from build123d import *

# Parameters (mm, degrees)
F0_W      = 45
F0_H      = 27
F0_R      = 1.5
F0_H_2    = 12
F1_DEPTH  = 8
F2_DEPTH  = 28
F3_R      = 1.5
F4_DEPTH  = 10
F5_DEPTH  = 8
F6_W      = 31
F6_H      = 12
F7_DEPTH  = 20
F8_SIZE2  = 19.5
F8_SIZE   = 20
F9_SIZE2  = 7.5
F9_SIZE   = 20
F11_DEPTH = 19.501
F12_DEPTH = 3
F13_R     = 7.7732339674
F14_DEPTH = 3
F16_DEPTH = 10
F17_DEPTH = 8
F18_R     = 1.5
F19_DEPTH = 16


with BuildPart() as f1:
    # F0 (on Top) → F1 (new body)
    with BuildSketch(Plane.XY):
        Rectangle(F0_W, F0_H)
        with Locations((-10, -10)):
            Circle(F0_R, mode=Mode.SUBTRACT)
        with Locations((10, -10)):
            Circle(F0_R, mode=Mode.SUBTRACT)
        with Locations((-10, 10)):
            Circle(F0_R, mode=Mode.SUBTRACT)
        with Locations((10, 10)):
            Circle(F0_R, mode=Mode.SUBTRACT)
        with Locations((0, 19.5)):
            Rectangle(F0_W, F0_H_2)
        with Locations((-10, 22)):
            Circle(F0_R, mode=Mode.SUBTRACT)
        with Locations((10, 22)):
            Circle(F0_R, mode=Mode.SUBTRACT)
    extrude(amount=F1_DEPTH)

    # F0 (on Top) → F2 (join)
    with BuildSketch(Plane.XY):
        with Locations((0, 19.5)):
            Rectangle(F0_W, F0_H_2)
        with Locations((-10, 22)):
            Circle(F0_R, mode=Mode.SUBTRACT)
        with Locations((10, 22)):
            Circle(F0_R, mode=Mode.SUBTRACT)
    extrude(amount=-F2_DEPTH)

    # F3 (on face) → F4 (cut)
    with BuildSketch(Plane(origin=(0, 0, -28), x_dir=(1, 0, 0), z_dir=(0, 0, -1))):
        Polygon((-7.25, -20.4122867597), (-10, -18.8245735195), (-12.75, -20.4122867597), (-12.75, -23.5877132403), (-12.75, -25.5), (-7.25, -25.5), (-7.25, -23.5877132403), align=None)
        with Locations((-10, -22)):
            Circle(F3_R, mode=Mode.SUBTRACT)
        Polygon((7.25, -23.5877132403), (7.25, -25.5), (12.75, -25.5), (12.75, -23.5877132403), (12.75, -20.4122867597), (10, -18.8245735195), (7.25, -20.4122867597), align=None)
        with Locations((10, -22)):
            Circle(F3_R, mode=Mode.SUBTRACT)
    extrude(amount=-F4_DEPTH, mode=Mode.SUBTRACT)

    # F3 (on face) → F5 (join)
    with BuildSketch(Plane(origin=(0, 0, -28), x_dir=(1, 0, 0), z_dir=(0, 0, -1))):
        Polygon((7.25, -23.5877132403), (7.25, -25.5), (12.75, -25.5), (12.75, -23.5877132403), (12.75, -20.4122867597), (10, -18.8245735195), (7.25, -20.4122867597), align=None)
        with Locations((10, -22)):
            Circle(F3_R, mode=Mode.SUBTRACT)
        Polygon((-7.25, -20.4122867597), (-10, -18.8245735195), (-12.75, -20.4122867597), (-12.75, -23.5877132403), (-12.75, -25.5), (-7.25, -25.5), (-7.25, -23.5877132403), align=None)
        with Locations((-10, -22)):
            Circle(F3_R, mode=Mode.SUBTRACT)
    extrude(amount=-F5_DEPTH)

    # F6 (on face) → F7 (join)
    with BuildSketch(Plane.XY.offset(8)):
        Polygon((-22.5, 25.5), (-22.5, -13.5), (-15.5, -13.5), (-15.5, -6), (-15.5, 6), (-15.5, 25.5), align=None)
        Rectangle(F6_W, F6_H)
        Polygon((15.5, 6), (15.5, -6), (15.5, -13.5), (22.5, -13.5), (22.5, 25.5), (15.5, 25.5), align=None)
    extrude(amount=F7_DEPTH)

    # F8
    f8_edges = [f1.edges().sort_by_distance(p)[0] for p in [
        (-19, 25.5, 28),
        (19, 25.5, 28),
    ]]
    f8_side = f1.faces().sort_by_distance((0, 25.5, -5.719915))[0]
    chamfer(f8_edges, length=F8_SIZE, length2=F8_SIZE2, reference=f8_side)

    # F9
    f9_edges = [f1.edges().sort_by_distance(p)[0] for p in [
        (19, -13.5, 28),
        (-19, -13.5, 28),
    ]]
    f9_side = f1.faces().sort_by_distance((-21.97, -13.5, 14))[0]
    chamfer(f9_edges, length=F9_SIZE, length2=F9_SIZE2, reference=f9_side)

    # F10 (on face) → F11 (cut, through all)
    with BuildSketch(Plane(origin=(0, 6, 0), x_dir=(-1, 0, 0), z_dir=(0, 1, 0))):
        with BuildLine():
            Line((5.6568542495, 28), (-5.6568542495, 28))
            ThreePointArc((-5.6568542495, 28), (0, 24), (5.6568542495, 28))
        make_face()
    extrude(amount=-F11_DEPTH, mode=Mode.SUBTRACT)

    # F10 (on face) → F12 (cut)
    with BuildSketch(Plane(origin=(0, 6, 0), x_dir=(-1, 0, 0), z_dir=(0, 1, 0))):
        with BuildLine():
            Line((-5.6568542495, 28), (-7.7459666924, 28))
            ThreePointArc((-7.7459666924, 28), (0, 22), (7.7459666924, 28))
            Line((7.7459666924, 28), (5.6568542495, 28))
            ThreePointArc((5.6568542495, 28), (0, 24), (-5.6568542495, 28))
        make_face()
    extrude(amount=-F12_DEPTH, mode=Mode.SUBTRACT)

    # F13 (on face) → F14 (cut)
    with BuildSketch(Plane.XZ.offset(6)):
        with Locations((0, 30)):
            Circle(F13_R)
    extrude(amount=-F14_DEPTH, mode=Mode.SUBTRACT)

    # F15 (on face) → F16 (cut)
    with BuildSketch(Plane.XY.offset(28)):
        Polygon((-19.5877132403, -2.75), (-16.4122867597, -2.75), (-14.8245735195, 0), (-16.4122867597, 2.75), (-19.5877132403, 2.75), (-22.5, 2.75), (-22.5, -2.75), align=None)
        Polygon((14.8245735195, 0), (16.4122867597, -2.75), (19.5877132403, -2.75), (22.5, -2.75), (22.5, 2.75), (19.5877132403, 2.75), (16.4122867597, 2.75), align=None)
    extrude(amount=-F16_DEPTH, mode=Mode.SUBTRACT)

    # F15 (on face) → F17 (join)
    with BuildSketch(Plane.XY.offset(28)):
        Polygon((-19.5877132403, -2.75), (-16.4122867597, -2.75), (-14.8245735195, 0), (-16.4122867597, 2.75), (-19.5877132403, 2.75), (-22.5, 2.75), (-22.5, -2.75), align=None)
        Polygon((14.8245735195, 0), (16.4122867597, -2.75), (19.5877132403, -2.75), (22.5, -2.75), (22.5, 2.75), (19.5877132403, 2.75), (16.4122867597, 2.75), align=None)
    extrude(amount=-F17_DEPTH)

    # F18 (on face) → F19 (cut)
    with BuildSketch(Plane.XY.offset(28)):
        with Locations((-18, 0)):
            Circle(F18_R)
        with Locations((18, 0)):
            Circle(F18_R)
    extrude(amount=-F19_DEPTH, mode=Mode.SUBTRACT)


solid = f1.part
Could you check a few things on this model? Use its own coordinates, in mm. A direction names the side the tool comes from. Round coordinates to 2 decimals unless told otherwise and drop trailing zeros. Write each loop counter-clockwise with the first axis right and the second up, starting at its lowest first coordinate (ties: lowest second). Pieces come first, ordered by that corner, then holes. Notation, with made-up numbers: (62, 82.5) - (112, 82.5) arc R28 ccw to (112, 119.5) - close; hole circle Ø8 at (24.5, -14.5). An arc over 180 degrees is marked (long way). Put each result on its own line as item: value. Start each with the question number.
(1) I want a section at B-B, the plane z = 6.5. Please give me the cut outline in (x, y).
(2) For faces 4 (the flat face through (0.5, -3, 23.6)), 5 (the flat face through (15.63, 1.394, 19.014)), 6 (the flat face through (-15.63, -1.394, 19.014)), 7 (the flat face through (0.1, 3, 23.7)), which set-ups out of +Z, -Z, +X, -X, +Y, -Y let a thin tool reach every point of the face, with its end or its side?
(3) Will these pins go through, and if not, where does the flat tip stop? pin 1 (2.5 mm diameter, centred on x = -10, y = -10, fed in from +Z); pin 2 (3 mm diameter, centred on x = -13, y = -7, fed in from -Z); pin 3 (1 mm diameter, centred on x = -20, z = 18.5, fed in from -Y); pin 4 (3.5 mm diameter, centred on x = 10, y = 22, fed in from +Z).
(4) I need wall thicknesses on probe 1 along Z at (x, y) = (17, 2.5); probe 2 along Y at (x, z) = (10, 3.25); probe 3 along Y at (x, z) = (-6, -9). Which ranges of each line are inside material? Lowest first, please.
(5) I want a section at A-A, the plane y = -10. Please give me the cut outline in (x, z).
(6) I want a section at C-C, the plane y = -5. Please give me the cut outline in (x, z).
(7) I want a section at D-D, the plane z = -10. Please give me the cut outline in (x, y).
(8) Thinking about a two-plate mould opening in X: for faces 1 (the flat face through (15.5, 12, 13)), 2 (the flat face through (0, 25.5, -10)), 3 (the flat face through (-15.61, 1.36, 19.01)), which applies, released by +X, released by -X, zero draft, split by the parting line, or undercut?
Here are the results:
1. outline: (-22.5, -13.5) - (22.5, -13.5) - (22.5, 25.5) - (-22.5, 25.5) - close; hole circle Ø3 at (-10, -10); hole circle Ø3 at (-10, 10); hole circle Ø3 at (-10, 22); hole circle Ø3 at (10, -10); hole circle Ø3 at (10, 10); hole circle Ø3 at (10, 22)
2. face 4: +Z, -Y
2. face 5: +X
2. face 6: -X
2. face 7: +Z, +Y
3. pin 1: passes through
3. pin 2: stops at z = 0
3. pin 3: stops at y = -9.75
3. pin 4: stops at z = 8
4. probe 1: z = 0 to 18, 20 to 28
4. probe 2: y = -13.5 to -11.5, -8.5 to 8.5, 11.5 to 20.5, 23.5 to 25.5
4. probe 3: y = 13.5 to 25.5
5. outline: (-22.5, 0) - (-11.5, 0) - (-11.5, 8) - (-15.5, 8) - (-15.5, 17.33) - (-22.5, 17.33) - close; (-8.5, 0) - (8.5, 0) - (8.5, 8) - (-8.5, 8) - close; (11.5, 0) - (22.5, 0) - (22.5, 17.33) - (15.5, 17.33) - (15.5, 8) - (11.5, 8) - close
6. outline: (-22.5, 0) - (22.5, 0) - (22.5, 28) - (7.51, 28) arc R7.77 cw to (-7.51, 28) - (-22.5, 28) - close
7. outline: (-22.5, 13.5) - (22.5, 13.5) - (22.5, 25.5) - (-22.5, 25.5) - close; hole circle Ø3 at (-10, 22); hole circle Ø3 at (10, 22)
8. face 1: undercut
8. face 2: zero draft
8. face 3: released by -X
